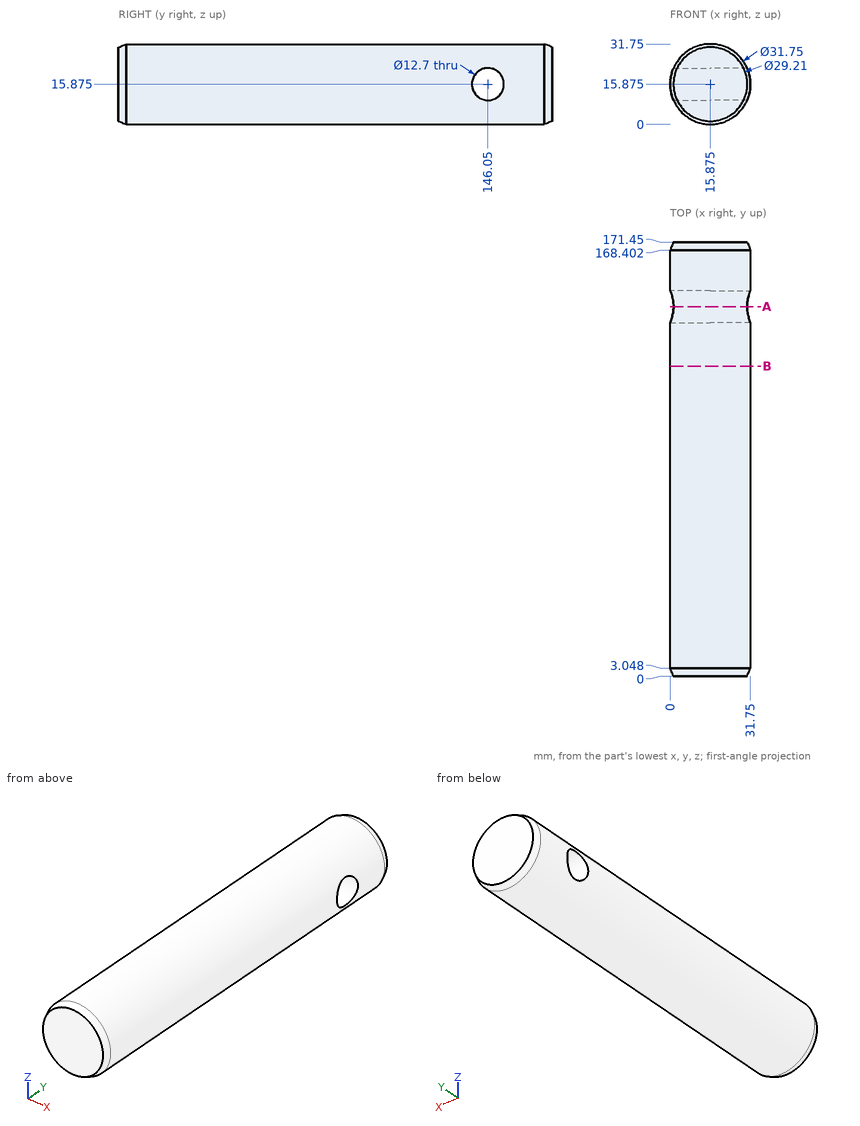
Verification items for this drawing (mm, ordinates from the low corner). Coordinates: 2 decimals unless noted, no trailing zeros. Loops run counter-clockwise (first coordinate to the right, second up) from the corner with the lowest first, then second, coordinate; pieces in that order, holes last. Notation, with made-up numbers: (-7, 33.25) -> (49, 33.25) arc R19 ccw to (49, 51.25) -> close; hole circle Ø8 at (59, -17.5). An arc over 180 degrees is marked (long way). Put each result on its own line as item: value.
1. Section check B-B, the plane y = 122.5. Record the boundary of the cut face in (x, z) (3 decimals), then the cut area to 3 significant figures.
Result set:
outline: circle Ø31.75 at (15.875, 15.875)
area: 792 mm^2
2. Gauge pin test, flat ends, axial feed: P1, Ø10, axis at y = 146.05, z = 15.875, coming from the -X side; P2, Ø5, axis at x = 27, y = 152, coming from the +Z side; P3, Ø2, axis at y = 46.5, z = 7, coming from the +X side; P4, Ø4, axis at x = 28, y = 62.5, coming from the -Z side. Record the tip position at first contact, or that the pin passes through.
Result set:
P1: passes through
P2: stops at z = 29.2
P3: stops at x = 29.66
P4: stops at z = 3.65
3. Thickness scan on line 1 (Y direction, x = 4, z = 10); line 2 (Z direction, x = 4, y = 146); line 3 (Z direction, x = 5.75, y = 146.05) (3 decimals). Record the ranges inside material, lowest first.
Result set:
line 1: y = 0 to 143.64, 148.46 to 171.45
line 2: z = 5.34 to 9.53, 22.22 to 26.41
line 3: z = 3.648 to 9.525, 22.225 to 28.102
4. Section check A-A, the plane y = 146.05. Record the boundary of the cut face in (x, z) (3 decimals).
Result set:
outline: (1.325, 9.525) arc R15.875 ccw to (30.425, 9.525) -> close; (1.325, 22.225) -> (30.425, 22.225) arc R15.875 ccw to start
